```python
from build123d import *

# Parameters (mm, degrees)
SKETCH1_R           = 44.45
SKETCH1_R_2         = 38.9763
BOSS_EXTRUDE1_DEPTH = 90
CAVITY1_START       = -6.35
CAVITY1_DEPTH       = 12.7
CAVITY1_2_DEPTH     = 12.7


# Read off the part's stored shape, not the designer's step: Cavity1
with BuildPart() as part:
    # Sketch1 → Boss-Extrude1 (new body)
    with BuildSketch(Plane.XY):
        with Locations(Location((0, 0, 0), (0, 0, 180))):
            Circle(SKETCH1_R)
        with Locations(Location((0, 0, 0), (0, 0, 180))):
            Circle(SKETCH1_R_2, mode=Mode.SUBTRACT)
    extrude(amount=BOSS_EXTRUDE1_DEPTH)

    # Cavity1 outline → Cavity1 (cut)
    with BuildSketch(Plane(origin=(0, 0, 0), x_dir=(-0.258888878578149, 0.9659071117600018, 0), z_dir=(0.9659071117600018, 0.25888887857814896, 0)).offset(CAVITY1_START)):
        with BuildLine():
            ThreePointArc((38.455551767, 70.863594779), (41.461594511, 71.680385005), (44.450315107, 72.558444487))
            Line((44.450315107, 72.558444487), (46, 73.030985488))
            Line((46, 73.030985488), (46, 90))
            Line((46, 90), (-46, 90))
            Line((-46, 90), (-46, 73.030985488))
            Line((-46, 73.030985488), (-44.450315107, 72.558444487))
            ThreePointArc((-44.450315107, 72.558444487), (-41.461594511, 71.680385005), (-38.455551767, 70.863594779))
            Line((-38.455551767, 70.863594779), (-31.309084293, 69))
            Line((-31.309084293, 69), (31.309084293, 69))
            Line((31.309084293, 69), (38.455551767, 70.863594779))
        make_face()
    extrude(amount=CAVITY1_DEPTH, mode=Mode.SUBTRACT)

    # Cavity1 2 outline → Cavity1 2 (cut)
    with BuildSketch(Plane(origin=(0, 0, 0), x_dir=(0.9659071117600018, 0.258888878578149, 0), z_dir=(0.25888887857814896, -0.9659071117600018, 0)).offset(CAVITY1_START)):
        with BuildLine():
            ThreePointArc((38.455551767, 70.863594779), (41.461594511, 71.680385005), (44.450315107, 72.558444487))
            Line((44.450315107, 72.558444487), (46, 73.030985488))
            Line((46, 73.030985488), (46, 90))
            Line((46, 90), (-46, 90))
            Line((-46, 90), (-46, 73.030985488))
            Line((-46, 73.030985488), (-44.450315107, 72.558444487))
            ThreePointArc((-44.450315107, 72.558444487), (-41.461594511, 71.680385005), (-38.455551767, 70.863594779))
            Line((-38.455551767, 70.863594779), (-31.309084293, 69))
            Line((-31.309084293, 69), (31.309084293, 69))
            Line((31.309084293, 69), (38.455551767, 70.863594779))
        make_face()
    extrude(amount=CAVITY1_2_DEPTH, mode=Mode.SUBTRACT)


solid = part.part
```
For this review, take the finished solid that the model builds, in its own axes (mm). A direction names the side the tool comes from. Coordinates: 2 decimals unless noted, no trailing zeros. Loops run counter-clockwise (first coordinate to the right, second up) from the corner with the lowest first, then second, coordinate; pieces in that order, holes last.
1. For line 1 (Y direction, x = 0, z = 33.5); line 2 (X direction, y = 4, z = 39.5); line 3 (Y direction, x = -30, z = 47), list the stretches that pass through material, from the lowest coordinate up.
2. Add section B-B, the plane z = 85.5. Give the boundary of the cut face in (x, y).
3. Add section D-D, the plane z = 41. Give the boundary of the cut face in (x, y).
4. Add section C-C, the plane y = 26.5. Give the boundary of the cut face in (x, z).
5. Insertion check: P1, Ø1, axis at y = -28.5, z = 54.5, coming from the -X side; P2, Ø1.5, axis at y = -23.5, z = 63.5, coming from the +X side; P3, Ø8, axis at x = -18.5, z = 32.5, coming from the -Y side. Each pin has a flat end and moves straight along its axis. Give the tip position at first contact, or say it passes through.
6. Mouldability with a two-part tool opening along Y and no side actions: class faces 1 (the flat face through (-38.213, -16.816, 80.566)), 2 (the flat face through (36, -20, 90)), 3 (the cylindrical face through (9.6, 43.4, 44.4)), 4 (the flat face through (38.138, 16.796, 80.566)) as +Y half, -Y half, draft (parallel to the pull), parting line (faces both ways), or undercut.
7. Add section A-A, the plane x = 0. Give the boundary of the cut face in (y, z).
8. For faces 5 (the cylindrical face through (10.66, -40.11, 71.69)), 6 (the flat face through (0.2, 39.3, 0)), list the 3-axis set-ups (+Z, -Z, +X, -X, +Y, -Y) from which the entire face can be reached by the end or side of a thin tool; tool diameter is ignored.
Result:
1. line 1: y = -44.45 to -38.98, 38.98 to 44.45
1. line 2: x = -44.27 to -38.77, 38.77 to 44.27
1. line 3: y = -32.8 to -24.88, 24.88 to 32.8
2. outline: (-44.14, -5.26) - (-38.79, -3.82) arc R38.98 cw to (-16.09, 35.5) - (-17.52, 40.85) arc R44.45 ccw to start; (-40.85, -17.52) arc R44.45 ccw to (5.26, -44.14) - (3.82, -38.79) arc R38.98 cw to (-35.5, -16.09) - close; (-5.26, 44.14) - (-3.82, 38.79) arc R38.98 cw to (35.5, 16.09) - (40.85, 17.52) arc R44.45 ccw to start; (16.09, -35.5) - (17.52, -40.85) arc R44.45 ccw to (44.14, 5.26) - (38.79, 3.82) arc R38.98 cw to start
3. outline: circle Ø88.9 at (0, 0); hole circle Ø77.95 at (0, 0)
4. outline: (-35.69, 0) - (-28.58, 0) - (-28.58, 90) - (-35.69, 90) - close; (28.58, 0) - (35.69, 0) - (35.69, 90) - (28.58, 90) - close
5. P1: stops at x = -34.52
5. P2: stops at x = 38.19
5. P3: stops at y = -42.02
6. face 1: undercut
6. face 2: draft
6. face 3: parting line
6. face 4: undercut
7. outline: (-44.45, 0) - (-38.98, 0) - (-38.98, 90) - (-44.45, 90) - close; (38.98, 0) - (44.45, 0) - (44.45, 90) - (38.98, 90) - close
8. face 5: +Z
8. face 6: -Z, +X, -X, +Y, -Y
